Can you work these out from the model? Positions are in its coordinate system, mm. A direction names the side the tool comes from. Round coordinates to 2 decimals unless told otherwise and drop trailing zeros. Loops run counter-clockwise (first coordinate to the right, second up) from the corner with the lowest first, then second, coordinate; pieces in that order, holes last. Notation, with made-up numbers: (15.25, 5.5) -> (67.25, 5.5) arc R14 ccw to (67.25, 9.5) -> close; hole circle Ø2 at (60, 53.25). An arc over 180 degrees is marked (long way). Answer as a JSON object with one key per item and string values.
```python
from build123d import *

# Parameters (mm, degrees)
F0_W         = 25
F0_H         = 30
F1_DEPTH     = 10
F2_R         = 1.5
F3_DEPTH     = 5
F4_R         = 2.5
F5_DEPTH     = 5
F6_R         = 2.5
F7_DEPTH     = 5
F8_W         = 6.5
F8_H         = 6
F9_DEPTH     = 7
F10_T1_DEPTH = 45
F11_R        = 2


# Not quite as in the source:
# - a fillet or chamfer that OpenCascade refuses, or shapes differently, is made with other operations: its cross-section is extruded or revolved along the edge and cut away or added


with BuildPart() as f1:
    # F0 (on Top) → F1 (new body)
    with BuildSketch(Plane.XY):
        Rectangle(F0_W, F0_H)
    extrude(amount=F1_DEPTH)

    # F2 (on face) → F3 (join)
    with BuildSketch(Plane(origin=(0, 15, 0), x_dir=(-1, 0, 0), z_dir=(0, 1, 0))):
        with Locations((0, 5)):
            Circle(F2_R)
    extrude(amount=F3_DEPTH)

    # F4 (on face) → F5 (cut)
    with BuildSketch(Plane.YZ.offset(12.5)):
        with Locations((7.5, 5)):
            Circle(F4_R)
    extrude(amount=-F5_DEPTH, mode=Mode.SUBTRACT)

    # F6 (on face) → F7 (cut)
    with BuildSketch(Plane(origin=(-12.5, 0, 0), x_dir=(0, -1, 0), z_dir=(-1, 0, 0))):
        with Locations((-7.5, 5)):
            Circle(F6_R)
    extrude(amount=-F7_DEPTH, mode=Mode.SUBTRACT)

    # F8 (on face) → F9 (cut)
    with BuildSketch(Plane.XZ.offset(15)):
        with Locations((7.25, 5)):
            Rectangle(F8_W, F8_H)
        with Locations((-7.25, 5)):
            Rectangle(F8_W, F8_H)
    extrude(amount=-F9_DEPTH, mode=Mode.SUBTRACT)

    # F10: fillet of radius 3 on 4 edges, made by hand

    # F10_s2 → F10_t1 (cut)
    with BuildSketch(Plane.XZ.offset(-22.5)):
        with BuildLine():
            ThreePointArc((-9.5, 10), (-11.6213203436, 9.1213203436), (-12.5, 7))
            Line((-12.5, 7), (-12.5, 10))
            Line((-12.5, 10), (-9.5, 10))
        make_face()
        with BuildLine():
            ThreePointArc((12.5, 7), (11.6213203436, 9.1213203436), (9.5, 10))
            Line((9.5, 10), (12.5, 10))
            Line((12.5, 10), (12.5, 7))
        make_face()
        with BuildLine():
            ThreePointArc((12.5, 3), (11.6213203436, 0.8786796564), (9.5, 0))
            Line((9.5, 0), (12.5, 0))
            Line((12.5, 0), (12.5, 3))
        make_face()
        with BuildLine():
            ThreePointArc((-9.5, 0), (-11.6213203436, 0.8786796564), (-12.5, 3))
            Line((-12.5, 3), (-12.5, 0))
            Line((-12.5, 0), (-9.5, 0))
        make_face()
    extrude(amount=F10_T1_DEPTH, mode=Mode.SUBTRACT)

    # F11
    f11_edges = [f1.edges().sort_by_distance(p)[0] for p in [
        (11.62132, 15, 0.87868),
        (12.5, 15, 5),
        (11.62132, 15, 9.12132),
        (0, 15, 0),
        (-11.62132, 15, 0.87868),
        (-12.5, 15, 5),
        (-11.62132, 15, 9.12132),
        (0, 15, 10),
    ]]
    fillet(f11_edges, radius=F11_R)


solid = f1.part
```
Q1. I want a section at D-D, the plane y = 2. Write out the boundary of the cut face in (x, z).
Determined:
{"outline": "(-12.5, 3) arc R3 ccw to (-9.5, 0) -> (9.5, 0) arc R3 ccw to (12.5, 3) -> (12.5, 7) arc R3 ccw to (9.5, 10) -> (-9.5, 10) arc R3 ccw to (-12.5, 7) -> close"}
Q2. I want a section at C-C, the plane x = 3. Write out the boundary of the cut face in (y, z), then the cut area to 3 significant figures.
Determined:
{"outline": "(-15, 0) -> (13, 0) arc R2 ccw to (15, 2) -> (15, 8) arc R2 ccw to (13, 10) -> (-15, 10) -> close", "area": "298 mm²"}
Q3. We'd pull the mould along Y, two halves only. Please class faces 4 (the flat face through (-7, -12, 2)), 5 (the cylindrical face through (-11.9, 14.43, 5.03)), 6 (the flat face through (-7.5, 8, 5)), 7 (the cylindrical face through (-10, 9, 7)): pulls with the +Y half, pulls with the -Y half, needs draft (parallel to the pull), parting line crosses it, or undercut.
Determined:
{"face 4": "needs draft", "face 5": "pulls with the +Y half", "face 6": "undercut", "face 7": "undercut"}
Q4. On a 3-axis mill with a long thin cutter (end or side, diameter ignored), from which of +Z, -Z, +X, -X, +Y, -Y can I reach the whole of each face in a straight line? I mean faces 1 (the flat face through (7, -8, 5)), 2 (the cylindrical face through (0.13, 14.43, 9.4)), 3 (the cylindrical face through (1.5, 17.46, 5.07)). Say none if no direction works.
Determined:
{"face 1": "-Y", "face 2": "+Z, +X, -X, +Y", "face 3": "+Y"}
Q5. I want a section at B-B, the plane y = -9. Write out the boundary of the cut face in (x, z), then the cut area to 3 significant figures.
Determined:
{"outline": "(-12.5, 3) arc R3 ccw to (-9.5, 0) -> (9.5, 0) arc R3 ccw to (12.5, 3) -> (12.5, 7) arc R3 ccw to (9.5, 10) -> (-9.5, 10) arc R3 ccw to (-12.5, 7) -> close; hole (-10.5, 2) -> (-4, 2) -> (-4, 8) -> (-10.5, 8) -> close; hole (4, 2) -> (10.5, 2) -> (10.5, 8) -> (4, 8) -> close", "area": "164 mm²"}
Q6. I want a section at A-A, the plane z = 5. Write out the boundary of the cut face in (x, y), then the cut area to 3 significant figures.
Determined:
{"outline": "(-12.5, -15) -> (-10.5, -15) -> (-10.5, -8) -> (-4, -8) -> (-4, -15) -> (4, -15) -> (4, -8) -> (10.5, -8) -> (10.5, -15) -> (12.5, -15) -> (12.5, 5) -> (7.5, 5) -> (7.5, 10) -> (12.5, 10) -> (12.5, 13) arc R2 ccw to (10.5, 15) -> (1.5, 15) -> (1.5, 20) -> (-1.5, 20) -> (-1.5, 15) -> (-10.5, 15) arc R2 ccw to (-12.5, 13) -> (-12.5, 10) -> (-7.5, 10) -> (-7.5, 5) -> (-12.5, 5) -> close", "area": "622 mm²"}
Q7. I'm going to push flat-ended pins straight in: pin 1 (3 mm diameter, centred on y = 7.5, z = 5, fed in from +X); pin 2 (2 mm diameter, centred on x = 6.5, z = 4.5, fed in from -Y); pin 3 (1.5 mm diameter, centred on y = 6.5, z = 5.5, fed in from -X). Where does each tip first touch, or does it pass through?
Determined:
{"pin 1": "x = 7.5", "pin 2": "y = -8", "pin 3": "x = -7.5"}
Q8. If I drill on L1, parallel to X at y = -10, z = 3.75; L2, parallel to Z at x = 9.5, y = -11.5; L3, parallel to Y at x = 9.5, z = 5, over which ranges is the centre line in solid material (lowest first)? Write a range as [from, to].
Determined:
{"L1": "[-12.5, -10.5], [-4, 4], [10.5, 12.5]", "L2": "[0, 2], [8, 10]", "L3": "[-8, 5], [10, 15]"}
